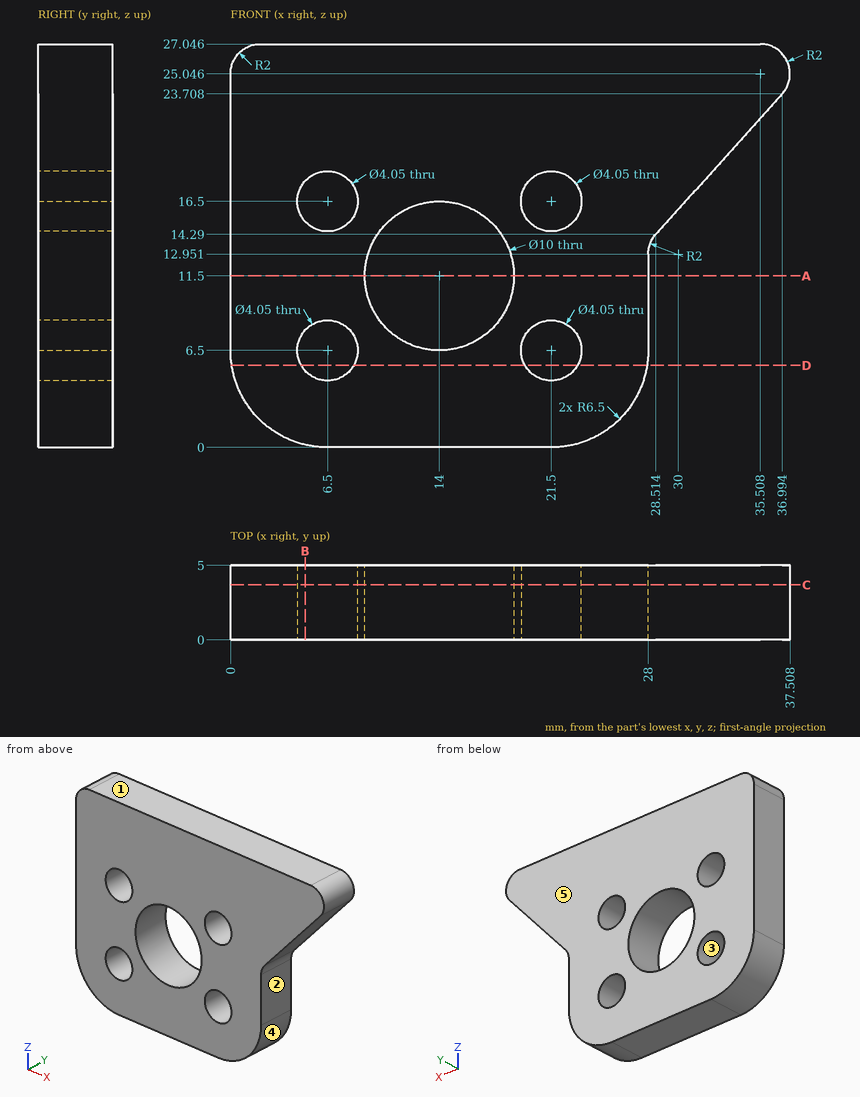
For this review, use the dimensioned drawing (mm, ordinates from the lowest corner) and the shaded views. A direction names the side the tool comes from. Round coordinates to 2 decimals unless told otherwise and drop trailing zeros. Write each loop counter-clockwise with the first axis right and the second up, starting at its lowest first coordinate (ties: lowest second). Pieces come first, ordered by that corner, then holes. Notation, with made-up numbers: (26, 40) - (80, 40) arc R36 ccw to (80, 74) - close; hole circle Ø8 at (68, 39). An arc over 180 degrees is marked (long way). One line per item, written item: value. Start each with the question number.
1. Consider section D-D on z = 5.5. Write out the cut boundary in (x, y).
2. To check wall thickness, follow L1, parallel to Z at x = 6.5, y = 3.9 (1 decimal); L2, parallel to Z at x = 14, y = 1.8; L3, parallel to X at y = 1.55, z = 11.5. State the ranges of each line that lie inside material, in increasing order. Write a range as from..to.
3. Consider section A-A on z = 11.5. Write out the cut boundary in (x, y).
4. Consider section C-C on y = 3.7. State how many separate pieces and enclosed holes the cut face has, and give its area (3 significant figures).
5. Consider section B-B on x = 5. Write out the cut boundary in (y, z) (1 decimal), and give its area (3 significant figures).
6. Machinability: for the marked faces 1 and 2, which of the approach directions +Z, -Z, +X, -X, +Y, -Y give a long, thin tool a straight path to every point of the face, cutting with its end or side? Answer none if there is none.
7. The part is to be moulded in two halves that separate along X. For the marked faces 3, 4 and 5, say which applies: released by +X, released by -X, zero draft, split by the parting line, or undercut.
Checks:
1. outline: (0.08, 0) - (4.74, 0) - (4.74, 5) - (0.08, 5) - close; (8.26, 0) - (19.74, 0) - (19.74, 5) - (8.26, 5) - close; (23.26, 0) - (27.92, 0) - (27.92, 5) - (23.26, 5) - close
2. L1: z = 0..4.5, 8.5..14.5, 18.5..27
2. L2: z = 0..6.5, 16.5..27.05
2. L3: x = 0..9, 19..28
3. outline: (0, 0) - (9, 0) - (9, 5) - (0, 5) - close; (19, 0) - (28, 0) - (28, 5) - (19, 5) - close
4. separate pieces: 1
4. enclosed holes: 5
4. area: 684 mm^2
5. outline: (0, 0.2) - (5, 0.2) - (5, 5.1) - (0, 5.1) - close; (0, 7.9) - (5, 7.9) - (5, 15.1) - (0, 15.1) - close; (0, 17.9) - (5, 17.9) - (5, 27) - (0, 27) - close
5. area: 107 mm^2
6. face 1: +Z, +X, -X, +Y, -Y
6. face 2: -Z, +X, +Y, -Y
7. face 3: undercut
7. face 4: released by +X
7. face 5: zero draft
